For this review, take the finished solid that the model builds, in its own axes (mm). A direction names the side the tool comes from. Coordinates: 2 decimals unless noted, no trailing zeros. Write each loop counter-clockwise with the first axis right and the second up, starting at its lowest first coordinate (ties: lowest second). Pieces come first, ordered by that corner, then holes. Notation, with made-up numbers: M -10.75,85.25 L 3.25,85.25 A25 cw 3.25,106.25 Z; hole C 41.25,32.5 d8. An arc over 180 degrees is marked long. Return JSON: item names as keys, results as strings.
```python
from build123d import *

# Parameters (mm, degrees)
BOX001_W     = 9.5
BOX001_H     = 7
BOX001_DEPTH = 3
SKETCH_W     = 8.981727
SKETCH_H     = 9.030207
SKETCH_R     = 1.530969
PAD_DEPTH    = 5


with BuildPart() as body044:
    # Box001 → Box001 (new body)
    with BuildSketch(Plane.XY):
        with Locations((4.75, 3.5)):
            Rectangle(BOX001_W, BOX001_H)
    extrude(amount=BOX001_DEPTH)


with BuildPart() as body044_1:
    # Body044 placement: moved
    add(body044.part.moved(Location((-4, -3.5, 1))))


with BuildPart() as cut005:
    # Sketch → Pad (new body)
    with BuildSketch(Plane.XY):
        with Locations((-0.03812, -0.019445)):
            Rectangle(SKETCH_W, SKETCH_H)
        Circle(SKETCH_R, mode=Mode.SUBTRACT)
    extrude(amount=PAD_DEPTH)

    # Cut005: cut Body044
    add(body044_1.part, mode=Mode.SUBTRACT)


with BuildPart() as cut005_1:
    # Cut005 placement: moved
    add(cut005.part.moved(Location((0, 0.025, 0))))


solid = cut005_1.part
```
1. Clearance check with flat-ended pins moving along their axes: pin 1 Ø1.8 at (x, y) = (0, 0.025) entering from +Z; pin 2 Ø1.5 at (y, z) = (2.5, 2.5) entering from +X. State where each tip first meets the part, or that it passes through.
Checks:
{"pin 1": "through", "pin 2": "x = -4"}
2. We need section C-C (z = 1.55). State the section outline as (x, y) points (3 decimals).
Checks:
{"outline": "M -4.529,-4.51 L 4.453,-4.51 L 4.453,-3.475 L -4,-3.475 L -4,3.525 L 4.453,3.525 L 4.453,4.521 L -4.529,4.521 Z"}
3. For faces 4 (the face through (0, 4.521, 2)), 5 (the face through (0, 2, 4)), list the 3-axis set-ups (+Z, -Z, +X, -X, +Y, -Y) from which the entire face can be reached by the end or side of a thin tool; tool diameter is ignored.
Checks:
{"face 4": "+Z, -Z, +X, -X, +Y", "face 5": "+X"}
4. Wall thickness on L1, parallel to Y at x = 0, z = 4.5; L2, parallel to Y at x = -3, z = 2.8 (3 decimals); L3, parallel to Z at x = 0.5, y = -3.25: over which ranges is each line inside the solid? List them lowest first. Write a range as from..to.
Checks:
{"L1": "-4.51..-1.51, 1.56..4.52", "L2": "-4.51..-3.475, 3.525..4.521", "L3": "0..1, 4..5"}
5. Draft analysis for pull direction Y (two halves, no side actions). For faces 1 (the face through (-1.21, -0.91, 4.49)), 2 (the face through (0, -4.51, 2)), 3 (the face through (4.453, -0.1, 0.8)), state which applies: +Y half, -Y half, draft (parallel to the pull), parting line (faces both ways), or undercut.
Checks:
{"face 1": "undercut", "face 2": "-Y half", "face 3": "draft"}
6. We need section D-D (x = 0). State the section outline as (y, z) points (3 decimals), plus the area to 3 significant figures.
Checks:
{"outline": "M -4.51,0 L -1.506,0 L -1.506,1 L -3.475,1 L -3.475,4 L -1.506,4 L -1.506,5 L -4.51,5 Z; M 1.556,0 L 4.521,0 L 4.521,5 L 1.556,5 L 1.556,4 L 3.525,4 L 3.525,1 L 1.556,1 Z", "area": "18.0 mm2"}
7. We need section A-A (x = 2.5). State the section outline as (y, z) points (3 decimals), plus the area to 3 significant figures.
Checks:
{"outline": "M -4.51,0 L 4.521,0 L 4.521,5 L -4.51,5 Z; hole M -3.475,1 L 3.525,1 L 3.525,4 L -3.475,4 Z", "area": "24.2 mm2"}
8. We need section B-B (y = -0.5). State the section outline as (x, z) points.
Checks:
{"outline": "M -4.53,0 L -1.44,0 L -1.44,1 L -4,1 L -4,4 L -1.44,4 L -1.44,5 L -4.53,5 Z; M 1.44,0 L 4.45,0 L 4.45,1 L 1.44,1 Z; M 1.44,4 L 4.45,4 L 4.45,5 L 1.44,5 Z"}
